Design review of the part built by this model. Coordinates are the model's own, in mm. Coordinates: 2 decimals unless noted, no trailing zeros. Write each loop counter-clockwise with the first axis right and the second up, starting at its lowest first coordinate (ties: lowest second). Pieces come first, ordered by that corner, then holes.
Q1. Take a section at D-D (x = 0). Give the boundary of the cut face in (y, z).
Q2. Take a section at B-B (x = 4.5). Give the boundary of the cut face in (y, z).
Q3. Mouldability with a two-part tool opening along X and no side actions: class faces 1 (the cylindrical face through (-6.943, 0.986, -0.891)), 2 (the flat face through (-2.1, 0, -5.3)), 3 (the cylindrical face through (-2.096, 1.014, 6.633)), 4 (the cylindrical face through (2.055, 1.014, 6.614)) as pulls with the +X half, pulls with the -X half, needs draft (parallel to the pull), parting line crosses it, or undercut.
Q4. Insertion check: pin 1 (1 mm diameter, centred on y = 1, z = -6, fed in from -X). The pin has a flat end and moves straight along its axis. Give the tip position at first contact, or say it passes through.
Q5. Take a section at A-A (z = 0). Give the boundary of the cut face in (x, y).
Q6. For probe 1 along X at (y, z) = (1.2, 0); probe 2 along Z at (x, y) = (0, 1.6); probe 3 along X at (y, z) = (1.1, 4), list the stretches that pass through material, from the lowest coordinate up.
Q7. Take a section at C-C (y = 1.25). Give the boundary of the cut face in (x, z).
```python
from build123d import *

# Parameters (mm, degrees)
SKETCH1_R           = 7
BOSS_EXTRUDE1_DEPTH = 2
SKETCH2_R           = 5.5
CUT_EXTRUDE1_DEPTH  = 2
SKETCH3_R           = 2.5
BOSS_EXTRUDE4_DEPTH = 2
SKETCH4_W           = 5
SKETCH4_H           = 5.341067824
CUT_EXTRUDE4_DEPTH  = 2
SKETCH6_R           = 1
BOSS_EXTRUDE6_DEPTH = 2
SKETCH8_R           = 1
BOSS_EXTRUDE7_DEPTH = 2
SKETCH9_R           = 5.5
CUT_EXTRUDE5_DEPTH  = 2


with BuildPart() as part:
    # Sketch1 → Boss-Extrude1 (new body)
    with BuildSketch(Plane(origin=(0, 0, 0), x_dir=(1, 0, 0), z_dir=(0, 1, 0))):
        with Locations(Location((0, 0, 0), (0, 0, 270))):
            Circle(SKETCH1_R)
    extrude(amount=BOSS_EXTRUDE1_DEPTH)

    # Sketch2 → Cut-Extrude1 (cut)
    with BuildSketch(Plane(origin=(0, 2, 0), x_dir=(1, 0, 0), z_dir=(0, 1, 0))):
        with Locations(Location((0, 0, 0), (0, 0, 270))):
            Circle(SKETCH2_R)
    extrude(amount=-CUT_EXTRUDE1_DEPTH, mode=Mode.SUBTRACT)

    # Sketch3 → Boss-Extrude4 (add)
    with BuildSketch(Plane.XZ):
        with Locations((0, -8.225966767)):
            Circle(SKETCH3_R)
    extrude(amount=-BOSS_EXTRUDE4_DEPTH)

    # Sketch4 → Cut-Extrude4 (cut)
    with BuildSketch(Plane(origin=(0, 2, 0), x_dir=(1, 0, 0), z_dir=(0, 1, 0))):
        with Locations((0, -7)):
            Rectangle(SKETCH4_W, SKETCH4_H)
    extrude(amount=-CUT_EXTRUDE4_DEPTH, mode=Mode.SUBTRACT)

    # Sketch6 → Boss-Extrude6 (add)
    with BuildSketch(Plane(origin=(0, 2, 0), x_dir=(1, 0, 0), z_dir=(0, 1, 0))):
        with Locations((2.5, -5.71866395)):
            Circle(SKETCH6_R)
    extrude(amount=-BOSS_EXTRUDE6_DEPTH)

    # Sketch8 → Boss-Extrude7 (add)
    with BuildSketch(Plane(origin=(0, 2, 0), x_dir=(1, 0, 0), z_dir=(0, 1, 0))):
        with Locations((-2.5, -5.71866395)):
            Circle(SKETCH8_R)
    extrude(amount=-BOSS_EXTRUDE7_DEPTH)

    # Sketch9 → Cut-Extrude5 (cut)
    with BuildSketch(Plane(origin=(0, 2, 0), x_dir=(1, 0, 0), z_dir=(0, 1, 0))):
        Circle(SKETCH9_R)
    extrude(amount=-CUT_EXTRUDE5_DEPTH, mode=Mode.SUBTRACT)


solid = part.part
```
Response:
1. outline: (0, -10.73) - (2, -10.73) - (2, -5.5) - (0, -5.5) - close
2. outline: (0, -5.36) - (2, -5.36) - (2, -3.16) - (0, -3.16) - close; (0, 3.16) - (2, 3.16) - (2, 5.36) - (0, 5.36) - close
3. face 1: pulls with the -X half
3. face 2: needs draft
3. face 3: undercut
3. face 4: undercut
4. pin 1: stops at x = -4.33
5. outline: (-7, 0) - (-5.5, 0) - (-5.5, 2) - (-7, 2) - close; (5.5, 0) - (7, 0) - (7, 2) - (5.5, 2) - close
6. probe 1: x = -7 to -5.5, 5.5 to 7
6. probe 2: z = -10.73 to -5.5
6. probe 3: x = -5.74 to -3.77, 3.77 to 5.74
7. outline: (-3.42, 6.11) arc R7 ccw to (-1.99, -6.71) arc R2.5 ccw (long way) to (1.99, -6.71) arc R7 ccw to (3.42, 6.11) arc R1 ccw (long way) to (1.61, 5.26) arc R5.5 cw (long way) to (-1.61, 5.26) arc R1 ccw (long way) to start
